Geometry check sheet. Reference: the model listing, model coordinates, mm. Give positions to 0.01 mm unless a question says otherwise; leave off trailing zeros. Loops run counter-clockwise (first coordinate to the right, second up) from the corner with the lowest first, then second, coordinate; pieces in that order, holes last. Notation, with made-up numbers: (11.5, -33.5) -> (68.5, -33.5) arc R11 cw to (68.5, -29.5) -> close; hole circle Ø5 at (36.5, -15.5). An arc over 180 degrees is marked (long way). Write each question's results on one line, items separated by ' | '. Start each with the question number.
1) Sectioned sample at D-D on z = 8. Count the separate pieces of the cut face and the enclosed holes in it, then the cut area to 4 significant figures.
2) Draft check along Y on faces 1 (the face through (1, 5, 5.54)), 2 (the face through (1, 5, 3)), 3 (the face through (1, 11.43, 4)), 4 (the face through (-1.259, 8, 4)). Enter one of: pulls with the +Y half, pulls with the -Y half, needs draft (parallel to the pull), parting line crosses it, or undercut.
3) Depth check by flat-ended pin: pin 1 (2 mm diameter, centred on y = 8, z = 1.5, fed in from -X) (3 decimals). Enter the tip coordinate at first touch or a pass-through.
4) Sectioned sample at B-B on x = 3.55. Record the cut outline in (y, z), then the cut area to 3 significant figures.
5) Scan lines: line 1 (Y direction, x = 0, z = 2.5) (3 decimals); line 2 (Z direction, x = 3.65, y = 5.25); line 3 (Y direction, x = -0.95, z = 3.75). Record each from-to range of solid material in increasing order. Write a range as from..to.
6) Sectioned sample at C-C on y = 3. Record the cut outline in (x, z).
```python
from build123d import *

# Parameters (mm, degrees)
BOSS_EXTRUDE1_DEPTH = 12
LPATTERN1_COUNT     = 2
LPATTERN1_PITCH     = 2.54
BOSS_EXTRUDE2_DEPTH = 2.54
LPATTERN2_COUNT     = 5
LPATTERN2_PITCH     = 2.54


with BuildPart() as part:
    # Sketch1 → Boss-Extrude1 (new body)
    with BuildSketch(Plane.XY):
        Polygon((-0.125, 0.225), (-0.225, 0.125), (-0.225, -0.125), (-0.125, -0.225), (0.125, -0.225), (0.225, -0.125), (0.225, 0.125), (0.125, 0.225), align=None)
    extrude(amount=BOSS_EXTRUDE1_DEPTH)


with BuildPart() as lpattern1_1:
    # LPattern1: pattern copy
    add(part.part.moved(Location(Vector(1, 0, 0) * (1 * LPATTERN1_PITCH))))


with BuildPart() as part_1:
    add(part.part)

    add(lpattern1_1.part)  # Boss-Extrude2 merges LPattern1_1
    # Sketch3 → Boss-Extrude2 (add)
    with BuildSketch(Plane(origin=(0, 0, 3), x_dir=(-1, 0, 0), z_dir=(0, 0, -1))):
        Polygon((-3.321218719, -1.27), (-3.821218719, -0.77), (-3.821218719, 0.77), (-3.321218719, 1.27), (0.758781281, 1.27), (1.258781281, 0.77), (1.258781281, -0.77), (0.758781281, -1.27), align=None)
    extrude(amount=-BOSS_EXTRUDE2_DEPTH)


with BuildPart() as lpattern2_1:
    # LPattern2: pattern copy
    add(part_1.part.moved(Location(Vector(0, 1, 0) * (1 * LPATTERN2_PITCH))))


with BuildPart() as lpattern2_2:
    # LPattern2: pattern copy
    add(part_1.part.moved(Location(Vector(0, 1, 0) * (2 * LPATTERN2_PITCH))))


with BuildPart() as lpattern2_3:
    # LPattern2: pattern copy
    add(part_1.part.moved(Location(Vector(0, 1, 0) * (3 * LPATTERN2_PITCH))))


with BuildPart() as lpattern2_4:
    # LPattern2: pattern copy
    add(part_1.part.moved(Location(Vector(0, 1, 0) * (4 * LPATTERN2_PITCH))))


with BuildPart() as part_2:
    add(part_1.part)

    # Combine1: union LPattern2_1, LPattern2_2, LPattern2_3, LPattern2_4
    add(lpattern2_1.part)
    add(lpattern2_2.part)
    add(lpattern2_3.part)
    add(lpattern2_4.part)


solid = part_2.part
```
Result:
1) separate pieces: 10 | enclosed holes: 0 | area: 1.825 mm^2
2) face 1: undercut | face 2: undercut | face 3: pulls with the +Y half | face 4: needs draft
3) pin 1: x = -0.225
4) outline: (-1.04, 3) -> (1.04, 3) -> (1.04, 5.54) -> (-1.04, 5.54) -> close; (1.5, 3) -> (3.58, 3) -> (3.58, 5.54) -> (1.5, 5.54) -> close; (4.04, 3) -> (6.12, 3) -> (6.12, 5.54) -> (4.04, 5.54) -> close; (6.58, 3) -> (8.66, 3) -> (8.66, 5.54) -> (6.58, 5.54) -> close; (9.12, 3) -> (11.2, 3) -> (11.2, 5.54) -> (9.12, 5.54) -> close | area: 26.4 mm^2
5) line 1: -0.225..0.225, 2.315..2.765, 4.855..5.305, 7.395..7.845, 9.935..10.385 | line 2: 3..5.54 | line 3: -1.08..1.08, 1.46..3.62, 4..6.16, 6.54..8.7, 9.08..11.24
6) outline: (-1.26, 3) -> (3.82, 3) -> (3.82, 5.54) -> (-1.26, 5.54) -> close
